Build history of the part. All positions in model axes, mm. A direction names the side the tool comes from. Round coordinates to 2 decimals unless told otherwise and drop trailing zeros. Loops run counter-clockwise (first coordinate to the right, second up) from the corner with the lowest first, then second, coordinate; pieces in that order, holes last. Notation, with made-up numbers: (27.5, 78) - (71.5, 78) arc R23 ccw to (71.5, 100) - close; hole circle Ø5 at (21.25, -21). An arc over 180 degrees is marked (long way). Use a Markdown table: item, result.
from build123d import *

# Parameters (mm, degrees)
F0_W     = 190.5
F0_H     = 19.05
F0_W_2   = 19.05
F0_H_2   = 12.7
F1_DEPTH = 9.525
F2_DEPTH = 9.525


with BuildPart() as f1:
    # F0 (on Top) → F1 (new body)
    with BuildSketch(Plane.XY):
        with Locations((-169.8625, 17.4625)):
            Rectangle(F0_W, F0_H)
        with Locations((-274.6375, 17.4625)):
            Rectangle(F0_W_2, F0_H)
        with Locations((-169.8625, -1.5875)):
            Rectangle(F0_W, F0_H)
        with Locations((-169.8625, -17.4625)):
            Rectangle(F0_W, F0_H_2)
        with Locations((-274.6375, -17.4625)):
            Rectangle(F0_W_2, F0_H_2)
        with Locations((-274.6375, -1.5875)):
            Rectangle(F0_W_2, F0_H)
        with Locations((-65.0875, 17.4625)):
            Rectangle(F0_W_2, F0_H)
        with Locations((-65.0875, -17.4625)):
            Rectangle(F0_W_2, F0_H_2)
        with Locations((-65.0875, -1.5875)):
            Rectangle(F0_W_2, F0_H)
    extrude(amount=F1_DEPTH)

    # F0 (on Top) → F2 (join)
    with BuildSketch(Plane.XY):
        with Locations((-169.8625, 17.4625)):
            Rectangle(F0_W, F0_H)
        with Locations((-169.8625, -17.4625)):
            Rectangle(F0_W, F0_H_2)
    extrude(amount=-F2_DEPTH)


solid = f1.part
Q1. Probe line 1 (Y direction, x = -170, z = -0.75); line 2 (X direction, y = 22, z = -8.25); line 3 (Z direction, x = -153.5, y = -7.5) (3 decimals). List the from-to ranges inside material, lowest first.
Results found:
| item | result |
|---|---|
| line 1 | y = -23.81 to -11.11, 7.94 to 26.99 |
| line 2 | x = -265.11 to -74.61 |
| line 3 | z = 0 to 9.525 |
Q2. Cut at A-A, the plane z = -5. List the corners of the cut face in (x, y).
Results found:
| item | result |
|---|---|
| outline | (-265.11, -23.81) - (-74.61, -23.81) - (-74.61, -11.11) - (-265.11, -11.11) - close; (-265.11, 7.94) - (-74.61, 7.94) - (-74.61, 26.99) - (-265.11, 26.99) - close |
Q3. Pull direction Y, two halves, no side cores. Call faces 1 (the face through (-265.112, 17, -5)), 2 (the face through (-171, 7.937, -5)), 3 (the face through (-168, 26.987, 0)): pulls with the +Y half, pulls with the -Y half, needs draft (parallel to the pull), parting line crosses it, or undercut.
Results found:
| item | result |
|---|---|
| face 1 | needs draft |
| face 2 | undercut |
| face 3 | pulls with the +Y half |
Q4. Cut at C-C, the plane x = -179.5. List the corners of the cut face in (y, z) (1 decimal).
Results found:
| item | result |
|---|---|
| outline | (-23.8, -9.5) - (-11.1, -9.5) - (-11.1, 0) - (7.9, 0) - (7.9, -9.5) - (27, -9.5) - (27, 9.5) - (-23.8, 9.5) - close |
Q5. Which spindle directions (+Z, -Z, +X, -X, +Y, -Y) get a long thin tool onto all of the face, cutting with end or side? Do faces 4 (the face through (-74.613, 17, -5)), 5 (the face through (-265.112, -18, -5)), 6 (the face through (-55.563, 1, 5)), 7 (the face through (-171, -11.112, -5)), 8 (the face through (-171, 2, 9.525)). Say none if no direction does.
Results found:
| item | result |
|---|---|
| face 4 | -Z, +X, +Y, -Y |
| face 5 | -Z, -X, +Y, -Y |
| face 6 | +Z, -Z, +X, +Y, -Y |
| face 7 | -Z, +X, -X |
| face 8 | +Z, +X, -X, +Y, -Y |
Q6. Drop flat-ended pins along their axis: pin 1 (5 mm diameter, centred on y = 18.5, z = -6, fed in from +X); pin 2 (4 mm diameter, centred on y = 11, z = -6, fed in from -X). Give the stop position or say it passes through.
Results found:
| item | result |
|---|---|
| pin 1 | stops at x = -74.61 |
| pin 2 | stops at x = -265.11 |
Q7. Cut at D-D, the plane y = -4. List the corners of the cut face in (x, z) (1 decimal).
Results found:
| item | result |
|---|---|
| outline | (-284.2, 0) - (-55.6, 0) - (-55.6, 9.5) - (-284.2, 9.5) - close |
Q8. Cut at B-B, the plane y = 15.5. List the corners of the cut face in (x, z) (1 decimal), plus the area to 3 significant figures.
Results found:
| item | result |
|---|---|
| outline | (-284.2, 0) - (-265.1, 0) - (-265.1, -9.5) - (-74.6, -9.5) - (-74.6, 0) - (-55.6, 0) - (-55.6, 9.5) - (-284.2, 9.5) - close |
| area | 3,990 mm2 |
